```python
from build123d import *

# Parameters (mm, degrees)
F0_W           = 55
F0_H           = 45
F1_DEPTH       = 15
F4_D           = 6
F4_DEPTH       = 15
F4_CSINK_D     = 10.4
F4_CSINK_ANGLE = 90
F4_TIP         = 1.8025818571
F5_D           = 5
F5_DEPTH       = 10
F5_TIP         = 1.5021515476


with BuildPart() as f1:
    # F0 (on Right) → F1 (new body)
    with BuildSketch(Plane.YZ):
        Rectangle(F0_W, F0_H)
    extrude(amount=F1_DEPTH)

    # F4
    with Locations(Plane(origin=(0, 0, 0), x_dir=(0, -1, 0), z_dir=(-1, 0, 0))):
        with Locations((-19.5, -14.5), (0, -14.5), (19.5, -14.5)):
            CounterSinkHole(F4_D / 2, F4_CSINK_D / 2, depth=F4_DEPTH, counter_sink_angle=F4_CSINK_ANGLE)
            with Locations((0, 0, -(F4_DEPTH + F4_TIP / 2))):  # 118° drill point
                Cone(0, F4_D / 2, F4_TIP, mode=Mode.SUBTRACT)

    # F5
    with Locations(Plane.YZ.offset(15)):
        with Locations((-17.5, 13.5), (17.5, 13.5)):
            Hole(F5_D / 2, depth=F5_DEPTH)
            with Locations((0, 0, -(F5_DEPTH + F5_TIP / 2))):  # 118° drill point
                Cone(0, F5_D / 2, F5_TIP, mode=Mode.SUBTRACT)


solid = f1.part
```
Could you check a few things on this model? Use its own coordinates, in mm. A direction names the side the tool comes from. Round coordinates to 2 decimals unless told otherwise and drop trailing zeros. Loops run counter-clockwise (first coordinate to the right, second up) from the corner with the lowest first, then second, coordinate; pieces in that order, holes last. Notation, with made-up numbers: M 58,15.5 L 62,15.5 A27 cw 62,36.5 Z; hole C 27,-1.75 d2. An arc over 180 degrees is marked long. Write item = value, one per line.
1. Thinking about a two-plate mould opening in Y: for faces 1 (the face through (7, 0, 22.5)), 2 (the face through (9.9, 19.5, 12)), 3 (the face through (7, -27.5, 0)), which applies, +Y half, -Y half, draft (parallel to the pull), parting line (faces both ways), or undercut?
Results below:
face_1 = draft
face_2 = undercut
face_3 = -Y half
2. I want a section at B-B, the plane z = -14.5. Write out the boundary of the cut face in (x, y), and give its area (3 significant figures).
Results below:
outline = M 0,-27.5 L 15,-27.5 L 15,-22.5 L 2.2,-22.5 L 0,-24.7 Z; M 0,-14.3 L 2.2,-16.5 L 15,-16.5 L 15,-3 L 2.2,-3 L 0,-5.2 Z; M 0,5.2 L 2.2,3 L 15,3 L 15,16.5 L 2.2,16.5 L 0,14.3 Z; M 0,24.7 L 2.2,22.5 L 15,22.5 L 15,27.5 L 0,27.5 Z
area = 540 mm²
3. I need wall thicknesses on probe 1 along Y at (x, z) = (11.25, 13.5); probe 2 along Z at (x, y) = (11.5, 0); probe 3 along Z at (x, y) = (12, 19.5). Which ranges of each line are inside material? Lowest first, please.
Results below:
probe_1 = -27.5 to -20, -15 to 15, 20 to 27.5
probe_2 = -22.5 to -17.5, -11.5 to 22.5
probe_3 = -22.5 to -17.5, -11.5 to 12, 15 to 22.5
4. I want a section at C-C, the plane y = 0. Write out the boundary of the cut face in (x, z), and give its area (3 significant figures).
Results below:
outline = M 0,-22.5 L 15,-22.5 L 15,-17.5 L 2.2,-17.5 L 0,-19.7 Z; M 0,-9.3 L 2.2,-11.5 L 15,-11.5 L 15,22.5 L 0,22.5 Z
area = 580 mm²
5. Will these pins go through, and if not, where does the flat tip stop? P1, Ø7, axis at y = 0, z = -14.5, coming from the -X side; P2, Ø8, axis at y = 19.5, z = -14.5, coming from the -X side.
Results below:
P1 = 1.7
P2 = 1.2
6. I want a section at A-A, the plane x = 13.5. Write out the boundary of the cut face in (y, z), and give its area (3 significant figures).
Results below:
outline = M -27.5,-22.5 L 27.5,-22.5 L 27.5,22.5 L -27.5,22.5 Z; hole C -19.5,-14.5 d6; hole C -17.5,13.5 d5; hole C 0,-14.5 d6; hole C 17.5,13.5 d5; hole C 19.5,-14.5 d6
area = 2,350 mm²
7. Which directions (+Z, -Z, +X, -X, +Y, -Y) give clear straight access to the entire face, cutting with the end or side of a thin tool? Please do faces 4 (the face through (2.09, 1.43, -17.26)), 5 (the face through (9.9, -15.5, 12)).
Results below:
face_4 = -X
face_5 = +X
